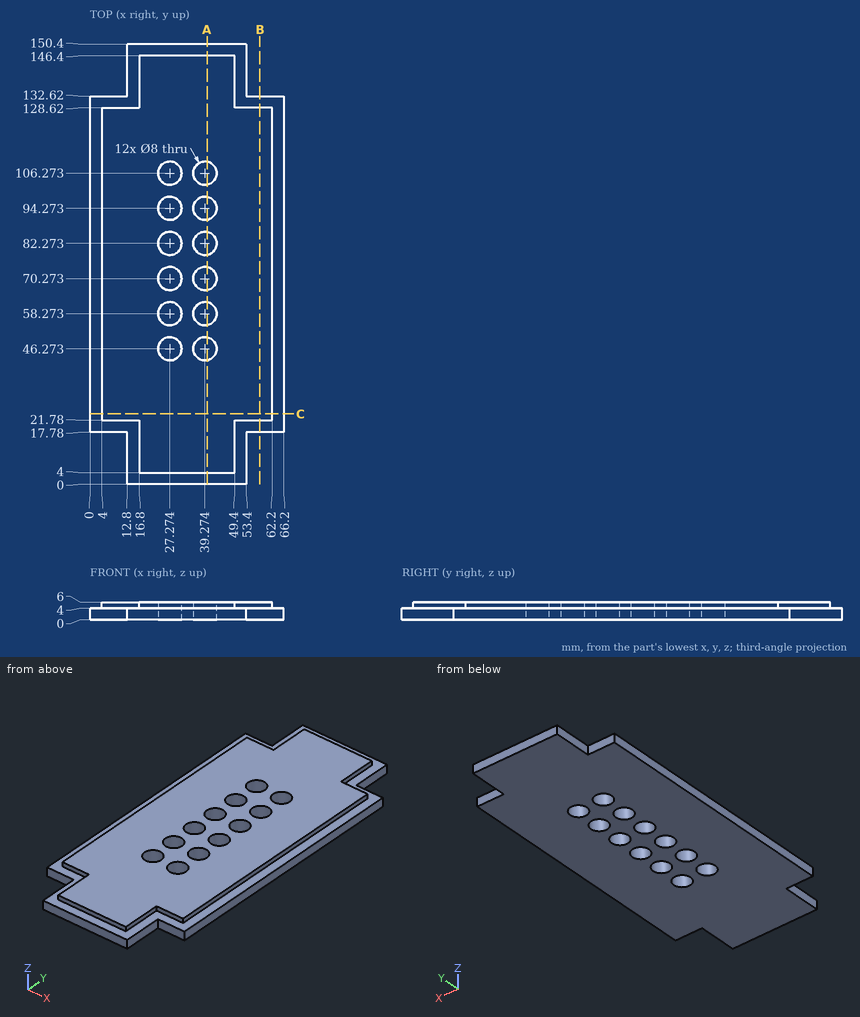
Drawing for the job (mm, zero at the part's lowest x, y, z). Give positions to 0.01 mm unless a question says otherwise; leave off trailing zeros. Order: outer loops, then holes, each group sorted by start corner. A loop starts at its lowest first (then second) coordinate and runs counter-clockwise, first axis right, second up. Notation, with made-up numbers: M -1.5,76.25 L 48.5,76.25 A22 cw 48.5,114.25 Z; hole C -5.5,-30.5 d9. An arc over 180 degrees is marked long. Put each result on its own line as item: value. Start each with the question number.
(1) Flat gauge pins, fed straight in: pin 1 Ø3 at (y, z) = (143, 3) entering from +X; pin 2 Ø2 at (x, y) = (29.5, 127.5) entering from -Z; pin 3 Ø3 at (x, z) = (62.5, 2.5) entering from -Y; pin 4 Ø5 at (x, y) = (39.27, 82.27) entering from +Z. Where does each tip first touch, or does it go through?
(2) Saw through at B-B, the plane x = 58. Write the cut outline in (y, z).
(3) Saw through at C-C, the plane y = 24. Write the cut outline in (x, z), then the cut area to 3 significant figures.
(4) Saw through at A-A, the plane x = 40. Give the number of separate pieces and of enclosed holes in the cut face, then the cut area to 3 significant figures.
(5) Drill centre lines: line 1 along X through (y, z) = (96.5, 2.8); line 2 along X through (y, z) = (107, 1.65); line 3 along X through (y, z) = (77, 5.2). Where is each one in solid material? Low to high.
Check result:
1. pin 1: stops at x = 53.4
1. pin 2: stops at z = 0
1. pin 3: stops at y = 17.78
1. pin 4: passes through
2. outline: M 17.78,0 L 132.62,0 L 132.62,4 L 128.62,4 L 128.62,6 L 21.78,6 L 21.78,4 L 17.78,4 Z
3. outline: M 0,0 L 66.2,0 L 66.2,4 L 62.2,4 L 62.2,6 L 4,6 L 4,4 L 0,4 Z
3. area: 381 mm2
4. separate pieces: 7
4. enclosed holes: 0
4. area: 603 mm2
5. line 1: x = 0 to 23.95, 30.6 to 35.95, 42.6 to 66.2
5. line 2: x = 0 to 23.34, 31.21 to 35.34, 43.21 to 66.2
5. line 3: x = 4 to 62.2
